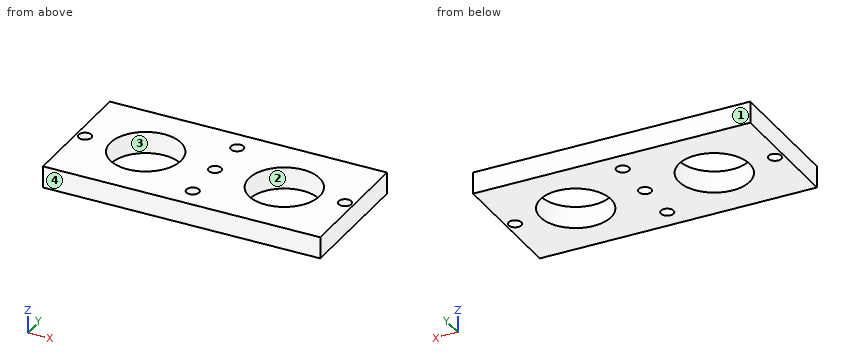
from build123d import *

# Parameters (mm, degrees)
SKETCH_1_W          = 64
SKETCH_1_H          = 30
SKETCH_1_R          = 8.16
EXTRUDE_1_DEPTH     = 5
SKETCH_2_R          = 1.45
CUT_EXTRUDE_1_DEPTH = 10


with BuildPart() as part:
    # 草图1 → 凸台-拉伸1 (new body)
    with BuildSketch(Plane.XY):
        with Locations((-6.884129186, 5.415137148)):
            Rectangle(SKETCH_1_W, SKETCH_1_H)
        with Locations((9.115870814, 5.415137148)):
            Circle(SKETCH_1_R, mode=Mode.SUBTRACT)
        with Locations((-22.884129186, 5.415137148)):
            Circle(SKETCH_1_R, mode=Mode.SUBTRACT)
    extrude(amount=EXTRUDE_1_DEPTH)

    # 草图2 → 切除-拉伸1 (cut)
    with BuildSketch(Plane.XY.offset(5)):
        with Locations((-6.884129186, 5.415137148)):
            Circle(SKETCH_2_R)
        with Locations((23.115870814, 5.415137148)):
            Circle(SKETCH_2_R)
        with Locations((-36.884129186, 5.415137148)):
            Circle(SKETCH_2_R)
        with Locations((-6.884129186, 15.415137148)):
            Circle(SKETCH_2_R)
        with Locations((-6.884129186, -4.584862852)):
            Circle(SKETCH_2_R)
    extrude(amount=-CUT_EXTRUDE_1_DEPTH, mode=Mode.SUBTRACT)


solid = part.part
Input: part model. Units: mm. Frame: model coordinates. Face numbers are marked on the shaded views. Round coordinates to 2 decimals unless told otherwise and drop trailing zeros. Write each loop counter-clockwise with the first axis right and the second up, starting at its lowest first coordinate (ties: lowest second). Pieces come first, ordered by that corner, then holes.
1) Ray query, L1, parallel to X at y = 5.25, z = 0.7; L2, parallel to X at y = 10.25, z = 2.75; L3, parallel to Y at x = -6, z = 0.55. Return the intervals inside material, ascending.
2) Cut plane D-D (z = 3.2). Return the cut outline in (x, y).
3) Cut plane B-B (x = -22.5). Return the cut outline in (y, z).
4) Cut plane A-A (y = 14.75). Return the cut outline in (x, z), then the cut area to 3 significant figures.
5) Contact query for a flat-ended pin moving along its axis: P1, Ø2.5, axis at x = -6.88, y = 15.42, coming from the +Z side. Output: stop coordinate, or through.
6) Draft query along Y for the marked faces 1, 2, 3 and 4. Return one class per face: pulls with the +Y half, pulls with the -Y half, needs draft (parallel to the pull), parting line crosses it, or undercut.
7) Cut plane C-C (y = -1.5). Return the cut outline in (x, z).
Geometry says:
1. L1: x = -38.88 to -38.32, -35.44 to -31.04, -14.73 to -8.32, -5.44 to 0.96, 17.27 to 21.68, 24.56 to 25.12
1. L2: x = -38.88 to -29.46, -16.31 to 2.54, 15.69 to 25.12
1. L3: y = -9.58 to -5.73, -3.44 to 4.27, 6.56 to 14.27, 16.56 to 20.42
2. outline: (-38.88, -9.58) - (25.12, -9.58) - (25.12, 20.42) - (-38.88, 20.42) - close; hole circle Ø2.9 at (-36.88, 5.42); hole circle Ø16.32 at (-22.88, 5.42); hole circle Ø2.9 at (-6.88, -4.58); hole circle Ø2.9 at (-6.88, 5.42); hole circle Ø2.9 at (-6.88, 15.42); hole circle Ø16.32 at (9.12, 5.42); hole circle Ø2.9 at (23.12, 5.42)
3. outline: (-9.58, 0) - (-2.74, 0) - (-2.74, 5) - (-9.58, 5) - close; (13.57, 0) - (20.42, 0) - (20.42, 5) - (13.57, 5) - close
4. outline: (-38.88, 0) - (-8.17, 0) - (-8.17, 5) - (-38.88, 5) - close; (-5.6, 0) - (25.12, 0) - (25.12, 5) - (-5.6, 5) - close
4. area: 307 mm2
5. P1: passes through
6. face 1: pulls with the +Y half
6. face 2: undercut
6. face 3: undercut
6. face 4: pulls with the -Y half
7. outline: (-38.88, 0) - (-27.22, 0) - (-27.22, 5) - (-38.88, 5) - close; (-18.55, 0) - (4.78, 0) - (4.78, 5) - (-18.55, 5) - close; (13.45, 0) - (25.12, 0) - (25.12, 5) - (13.45, 5) - close
